The model under review builds one solid part; all positions refer to its coordinate system, in mm. A direction names the side the tool comes from. Coordinates: 2 decimals unless noted, no trailing zeros. Order: outer loops, then holes, each group sorted by start corner. A loop starts at its lowest first (then second) coordinate and runs counter-clockwise, first axis right, second up. Notation, with made-up numbers: M 27.25,78.5 L 63.25,78.5 A13 cw 63.25,97.5 Z; hole C -4,26 d1. An arc over 180 degrees is marked long. Answer in a Markdown table with one row per item.
from build123d import *

# Parameters (mm, degrees)
SKETCH1_W           = 215.9
SKETCH1_H           = 42.333333334
BOSS_EXTRUDE1_DEPTH = 8.466666667
REAR_PIN_DEPTH      = 6.35
FRONT_PIN_DEPTH     = 6.35
TOP_PINS_DEPTH      = 6.35
PIN_CHAMFER_SIZE    = 0.635


with BuildPart() as part:
    # Sketch1 → Boss-Extrude1 (new body)
    with BuildSketch(Plane.XY):
        Rectangle(SKETCH1_W, SKETCH1_H)
        Polygon((-103.716666667, -12.7), (103.716666667, -12.7), (103.716666667, 5.604933333), (69.045666667, 5.604933333), (61.9506, 12.7), (-103.716666667, 12.7), align=None, mode=Mode.SUBTRACT)
    extrude(amount=BOSS_EXTRUDE1_DEPTH)

    # Sketch3 → rear pin (cut)
    with BuildSketch(Plane(origin=(-107.95, 0, 91.206646131), x_dir=(0, 0, -1), z_dir=(1, 0, 0))):
        Polygon((83.798312798, 16.933333333), (86.973312798, 20.108333333), (90.148312798, 16.933333333), (86.973312798, 13.758333333), align=None)
        Polygon((86.973312798, -20.108333333), (83.798312798, -16.933333333), (86.973312798, -13.758333333), (90.148312798, -16.933333333), align=None)
    extrude(amount=REAR_PIN_DEPTH, mode=Mode.SUBTRACT)

    # Sketch4 → front pin (cut)
    with BuildSketch(Plane(origin=(107.95, 0, 0), x_dir=(0, 0, -1), z_dir=(1, 0, 0))):
        Polygon((-1.058333333, 9.838266667), (-4.233333333, 13.013266667), (-7.408333333, 9.838266667), (-4.233333333, 6.663266667), align=None)
        Polygon((-1.058333333, -16.933333333), (-4.233333333, -13.758333333), (-7.408333333, -16.933333333), (-4.233333333, -20.108333333), align=None)
    extrude(amount=-FRONT_PIN_DEPTH, mode=Mode.SUBTRACT)

    # Sketch5 → top pins (cut)
    with BuildSketch(Plane(origin=(0, 21.166666667, 0), x_dir=(1, 0, 0), z_dir=(0, 1, 0))):
        Polygon((106.891666667, -4.233333333), (103.716666667, -7.408333333), (100.541666667, -4.233333333), (103.716666667, -1.058333333), align=None)
        Polygon((-3.175000085, -4.233333333), (-6.350000085, -7.408333333), (-9.525000085, -4.233333333), (-6.350000085, -1.058333333), align=None)
        Polygon((-15.875000085, -4.233333333), (-19.050000085, -7.408333333), (-22.225000085, -4.233333333), (-19.050000085, -1.058333333), align=None)
    extrude(amount=-TOP_PINS_DEPTH, mode=Mode.SUBTRACT)

    # pin chamfer
    pin_chamfer_edges = [part.edges().sort_by_distance(p)[0] for p in [
        (-4.762500085, 14.816666667, 2.645833333),
        (-4.762500085, 14.816666667, 5.820833333),
        (-7.937500085, 14.816666667, 5.820833333),
        (-7.937500085, 14.816666667, 2.645833333),
        (-4.762500085, 21.166666667, 2.645833333),
        (-7.937500085, 21.166666667, 2.645833333),
        (-7.937500085, 21.166666667, 5.820833333),
        (-4.762500085, 21.166666667, 5.820833333),
        (-17.462500085, 14.816666667, 2.645833333),
        (-17.462500085, 14.816666667, 5.820833333),
        (-20.637500085, 14.816666667, 5.820833333),
        (-20.637500085, 14.816666667, 2.645833333),
        (-17.462500085, 21.166666667, 2.645833333),
        (-20.637500085, 21.166666667, 2.645833333),
        (-20.637500085, 21.166666667, 5.820833333),
        (-17.462500085, 21.166666667, 5.820833333),
        (-107.95, 15.345833333, 5.820833333),
        (-107.95, 15.345833333, 2.645833333),
        (-107.95, 18.520833333, 2.645833333),
        (-107.95, 18.520833333, 5.820833333),
        (-101.6, 15.345833333, 5.820833333),
        (-101.6, 15.345833333, 2.645833333),
        (-101.6, 18.520833333, 2.645833333),
        (-101.6, 18.520833333, 5.820833333),
        (-107.95, -18.520833333, 2.645833333),
        (-107.95, -15.345833333, 2.645833333),
        (-107.95, -15.345833333, 5.820833333),
        (-107.95, -18.520833333, 5.820833333),
        (-101.6, -18.520833333, 2.645833333),
        (-101.6, -15.345833333, 2.645833333),
        (-101.6, -15.345833333, 5.820833333),
        (-101.6, -18.520833333, 5.820833333),
        (101.6, 8.250766667, 2.645833333),
        (101.6, 8.250766667, 5.820833333),
        (101.6, 11.425766667, 5.820833333),
        (101.6, 11.425766667, 2.645833333),
        (107.95, 8.250766667, 2.645833333),
        (107.95, 11.425766667, 2.645833333),
        (107.95, 11.425766667, 5.820833333),
        (107.95, 8.250766667, 5.820833333),
        (101.6, -18.520833333, 2.645833333),
        (101.6, -18.520833333, 5.820833333),
        (101.6, -15.345833333, 5.820833333),
        (101.6, -15.345833333, 2.645833333),
        (107.95, -18.520833333, 2.645833333),
        (107.95, -15.345833333, 2.645833333),
        (107.95, -15.345833333, 5.820833333),
        (107.95, -18.520833333, 5.820833333),
        (105.304166667, 14.816666667, 2.645833333),
        (105.304166667, 14.816666667, 5.820833333),
        (102.129166667, 14.816666667, 5.820833333),
        (102.129166667, 14.816666667, 2.645833333),
        (105.304166667, 21.166666667, 2.645833333),
        (102.129166667, 21.166666667, 2.645833333),
        (102.129166667, 21.166666667, 5.820833333),
        (105.304166667, 21.166666667, 5.820833333),
    ]]
    chamfer(pin_chamfer_edges, length=PIN_CHAMFER_SIZE)


solid = part.part
(1) To check wall thickness, follow line 1 (Y direction, x = -1.5, z = 0.5); line 2 (X direction, y = 16, z = 5) (3 decimals); line 3 (X direction, y = -1, z = 4.5). State the ranges of each line that lie inside material, in increasing order. Write a range as [from, to].
Report:
| item | result |
|---|---|
| line 1 | [-21.17, -12.7], [12.7, 21.17] |
| line 2 | [-101.6, -21.458], [-16.642, -8.758], [-3.942, 101.308], [106.125, 107.95] |
| line 3 | [-107.95, -103.72], [103.72, 107.95] |
(2) Take a section at A-A (y = 1). Write out the cut boundary in (x, z), then the cut area to 3 significant figures.
Report:
| item | result |
|---|---|
| outline | M -107.95,0 L -103.72,0 L -103.72,8.47 L -107.95,8.47 Z; M 103.72,0 L 107.95,0 L 107.95,8.47 L 103.72,8.47 Z |
| area | 71.7 mm^2 |
(3) Take a section at B-B (x = 74.5). Write out the cut boundary in (y, z).
Report:
| item | result |
|---|---|
| outline | M -21.17,0 L -12.7,0 L -12.7,8.47 L -21.17,8.47 Z; M 5.6,0 L 21.17,0 L 21.17,8.47 L 5.6,8.47 Z |
(4) Machinability: for faces 4 (the flat face through (-107.628, -18.771, 6.014)), 5 (the flat face through (-17.27, 20.84, 2.4)), 6 (the flat face through (65.55, 9.1, 4.17)), 7 (the flat face through (107.63, -18.77, 2.45)), which of the approach directions +Z, -Z, +X, -X, +Y, -Y give a long, thin tool a straight path to every point of the face, cutting with its end or side? Answer none if there is none.
Report:
| item | result |
|---|---|
| face 4 | -X |
| face 5 | +Y |
| face 6 | +Z, -Z |
| face 7 | +X |
(5) The part is to be moulded in two halves that separate along Y. For faces 1 (the flat face through (-2, -21.167, 4)), 2 (the flat face through (-20.83, 20.845, 6.071)), 3 (the flat face through (101.6, -17, 4)), say which applies: +Y half, -Y half, draft (parallel to the pull), parting line (faces both ways), or undercut.
Report:
| item | result |
|---|---|
| face 1 | -Y half |
| face 2 | +Y half |
| face 3 | undercut |
(6) Insertion check: P1, Ø3.5, axis at x = 103.5, z = 4, coming from the +Y side; P2, Ø3.5, axis at y = -17.5, z = 4.5, coming from the +X side; P3, Ø2.5, axis at y = 10.5, z = 4.5, coming from the +X side. Each pin has a flat end and moves straight along its axis. Give the tip position at first contact, or say it passes through.
Report:
| item | result |
|---|---|
| P1 | y = 15.27 |
| P2 | x = 107.41 |
| P3 | x = 101.9 |
